Could you check a few things on this model? Use its own coordinates, in mm. Give positions to 0.01 mm unless a question says otherwise; leave off trailing zeros. Loops run counter-clockwise (first coordinate to the right, second up) from the corner with the lowest first, then second, coordinate; pieces in that order, holes last. Notation, with made-up numbers: (-27, 15.25) - (-18, 15.25) arc R27 ccw to (-18, 52.25) - close; hole circle Ø4 at (48, 8.25). An arc over 180 degrees is marked (long way). Use CSV: the item, a comma, the result in double quotes.
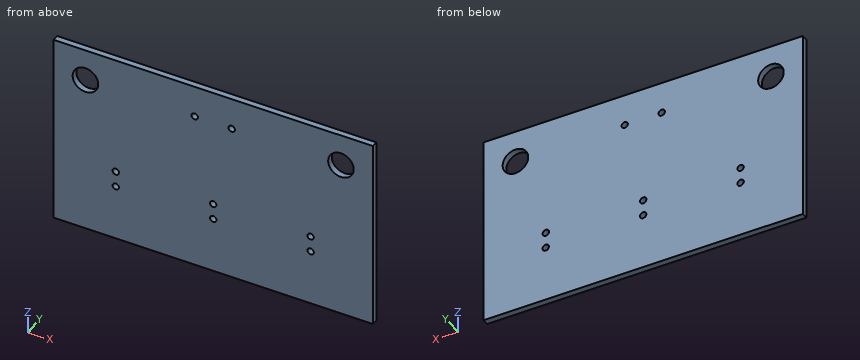
from build123d import *

# Parameters (mm, degrees)
SKETCH1_W           = 50
SKETCH1_H           = 30
BOSS_EXTRUDE1_DEPTH = 1
SKETCH2_R           = 0.5
SKETCH2_R_2         = 2
CUT_EXTRUDE1_DEPTH  = 1


with BuildPart() as part:
    # Sketch1 → Boss-Extrude1 (new body)
    with BuildSketch(Plane(origin=(0, 0, 0), x_dir=(1, 0, 0), z_dir=(0, 1, 0))):
        with Locations((25, 15)):
            Rectangle(SKETCH1_W, SKETCH1_H)
    extrude(amount=BOSS_EXTRUDE1_DEPTH)

    # Sketch2 → Cut-Extrude1 (cut)
    with BuildSketch(Plane(origin=(0, 1, 0), x_dir=(1, 0, 0), z_dir=(0, 1, 0))):
        with Locations((22.1, 5)):
            Circle(SKETCH2_R)
        with Locations((27.9, 5)):
            Circle(SKETCH2_R)
        with Locations((9.75, 18.75)):
            Circle(SKETCH2_R)
        with Locations((9.75, 21.25)):
            Circle(SKETCH2_R)
        with Locations((25, 18.75)):
            Circle(SKETCH2_R)
        with Locations((25, 21.25)):
            Circle(SKETCH2_R)
        with Locations((40.25, 18.75)):
            Circle(SKETCH2_R)
        with Locations((40.25, 21.25)):
            Circle(SKETCH2_R)
        with Locations((45, 5)):
            Circle(SKETCH2_R_2)
        with Locations((5, 5)):
            Circle(SKETCH2_R_2)
    extrude(amount=-CUT_EXTRUDE1_DEPTH, mode=Mode.SUBTRACT)


solid = part.part
1) Suppose I cut it at B-B (z = -5). Please give me the cut outline in (x, y), plus the area to 3 significant figures.
Answer below:
outline,"(0, 0) - (3, 0) - (3, 1) - (0, 1) - close; (7, 0) - (21.6, 0) - (21.6, 1) - (7, 1) - close; (22.6, 0) - (27.4, 0) - (27.4, 1) - (22.6, 1) - close; (28.4, 0) - (43, 0) - (43, 1) - (28.4, 1) - close; (47, 0) - (50, 0) - (50, 1) - (47, 1) - close"
area,"40.0 mm2"
2) Suppose I cut it at D-D (z = -21.25). Please give me the cut outline in (x, y).
Answer below:
outline,"(0, 0) - (9.25, 0) - (9.25, 1) - (0, 1) - close; (10.25, 0) - (24.5, 0) - (24.5, 1) - (10.25, 1) - close; (25.5, 0) - (39.75, 0) - (39.75, 1) - (25.5, 1) - close; (40.75, 0) - (50, 0) - (50, 1) - (40.75, 1) - close"
3) I'm going to push a flat-ended pin straight in: P1, Ø4.5, axis at x = 45, z = -5, coming from the +Y side. Where does the tip first touch, or does it pass through?
Answer below:
P1,"stops at y = 1"
4) I need wall thicknesses on line 1 along Z through (x, y) = (40.25, 0.5); line 2 along X through (y, z) = (0.4, -21.25); line 3 along Z through (x, y) = (22.1, 0.7). Which ranges of each line are inside material? Lowest first, please.
Answer below:
line 1,"z = -30 to -21.75, -20.75 to -19.25, -18.25 to 0"
line 2,"x = 0 to 9.25, 10.25 to 24.5, 25.5 to 39.75, 40.75 to 50"
line 3,"z = -30 to -5.5, -4.5 to 0"
5) Suppose I cut it at C-C (y = 0.5). State how many separate pieces and enclosed holes the cut face has, plus the area to 3 significant figures.
Answer below:
separate pieces,"1"
enclosed holes,"10"
area,"1,470 mm2"
6) Suppose I cut it at A-A (x = 40.25). Please give me the cut outline in (y, z).
Answer below:
outline,"(0, -30) - (1, -30) - (1, -21.75) - (0, -21.75) - close; (0, -20.75) - (1, -20.75) - (1, -19.25) - (0, -19.25) - close; (0, -18.25) - (1, -18.25) - (1, 0) - (0, 0) - close"
